Answer from the drawing. Dimensions are ordinates in mm from the lowest x, y and z of the part. Round coordinates to 2 decimals unless told otherwise and drop trailing zeros. Order: outer loops, then holes, each group sorted by start corner. A loop starts at its lowest first (then second) coordinate and runs counter-clockwise, first axis right, second up. Notation, with made-up numbers: M 37,49.5 L 50,49.5 A11 cw 50,61.5 Z; hole C 29.25,33.25 d11. An arc over 180 degrees is marked long. Use one line per item in the form item = value. Start each with the question number.
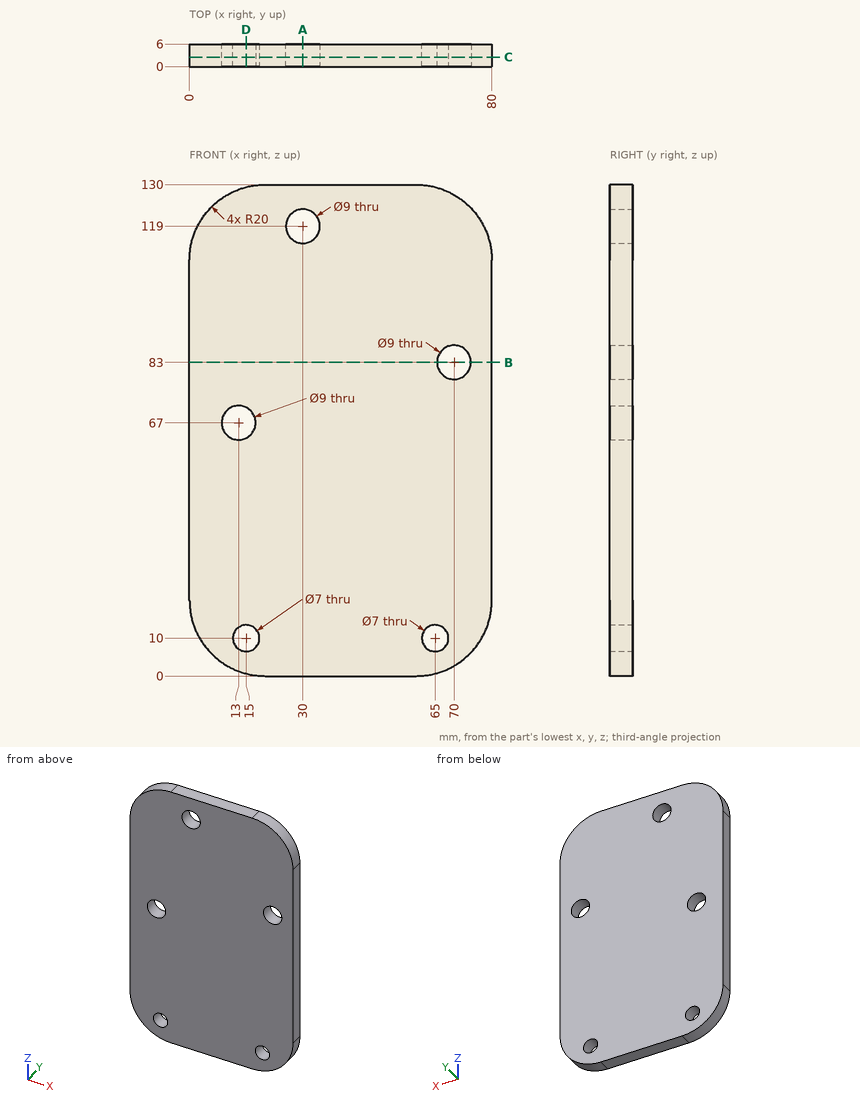
Item 1: Section A-A (x = 30) is taken. Write down the section's boundary in (y, z).
Item 2: Find the intervals of material crossed by L1, parallel to Z at x = 15, y = 2.65; L2, parallel to Z at x = 29.5, y = 4.75; L3, parallel to Z at x = 70, y = 3.2, in increasing order. Write a range as [from, to].
Item 3: Section D-D (x = 15) is taken. Write down the section's boundary in (y, z), and give its area (3 significant figures).
Item 4: Section C-C (y = 2.5) is taken. Write down the section's boundary in (x, z), and give its area (3 significant figures).
Item 5: Given P1, Ø9, axis at x = 15, z = 10, coming from the -Y side; P2, Ø2, axis at y = 5.5, z = 15.5, coming from the -X side; P3, Ø8, axis at x = 30, z = 119, coming from the -Y side; P4, Ø1.5, axis at x = 11, y = 2.5, coming from the -Z side, each flat-ended and moving along its own axis, determine where each tip first touches the part or whether it passes through.
Item 6: Section B-B (z = 83) is taken. Write down the section's boundary in (x, y), and give its area (3 significant figures).
The answers:
q1.outline = M 0,0 L 6,0 L 6,114.5 L 0,114.5 Z; M 0,123.5 L 6,123.5 L 6,130 L 0,130 Z
q2.L1 = [0.64, 6.5], [13.5, 62.97], [71.03, 129.36]
q2.L2 = [0, 114.53], [123.47, 130]
q2.L3 = [2.68, 78.5], [87.5, 127.32]
q3.outline = M 0,0.64 L 6,0.64 L 6,6.5 L 0,6.5 Z; M 0,13.5 L 6,13.5 L 6,62.97 L 0,62.97 Z; M 0,71.03 L 6,71.03 L 6,129.36 L 0,129.36 Z
q3.area = 682 mm²
q4.outline = M 0,20 A20 ccw 20,0 L 60,0 A20 ccw 80,20 L 80,110 A20 ccw 60,130 L 20,130 A20 ccw 0,110 Z; hole C 13,67 d9; hole C 15,10 d7; hole C 30,119 d9; hole C 65,10 d7; hole C 70,83 d9
q4.area = 9,790 mm²
q5.P1 = 0
q5.P2 = 0.31
q5.P3 = through
q5.P4 = 1.78
q6.outline = M 0,0 L 65.5,0 L 65.5,6 L 0,6 Z; M 74.5,0 L 80,0 L 80,6 L 74.5,6 Z
q6.area = 426 mm²
